The figure shows three views and two pictorial views of one solid part (mm, origin at its lowest corner). Answer the questions. A direction names the side the tool comes from. Coordinates: 2 decimals unless noted, no trailing zeros. Order: outer loops, then holes, each group sorted by start corner. A loop starts at its lowest first (then second) coordinate and runs counter-clockwise, first axis right, second up. Notation, with made-up numbers: M 12,79.25 L 71,79.25 A24 ccw 71,99.25 Z; hole C 27,-15.75 d2. An arc over 180 degrees is marked long. Use a Markdown table: item, result.
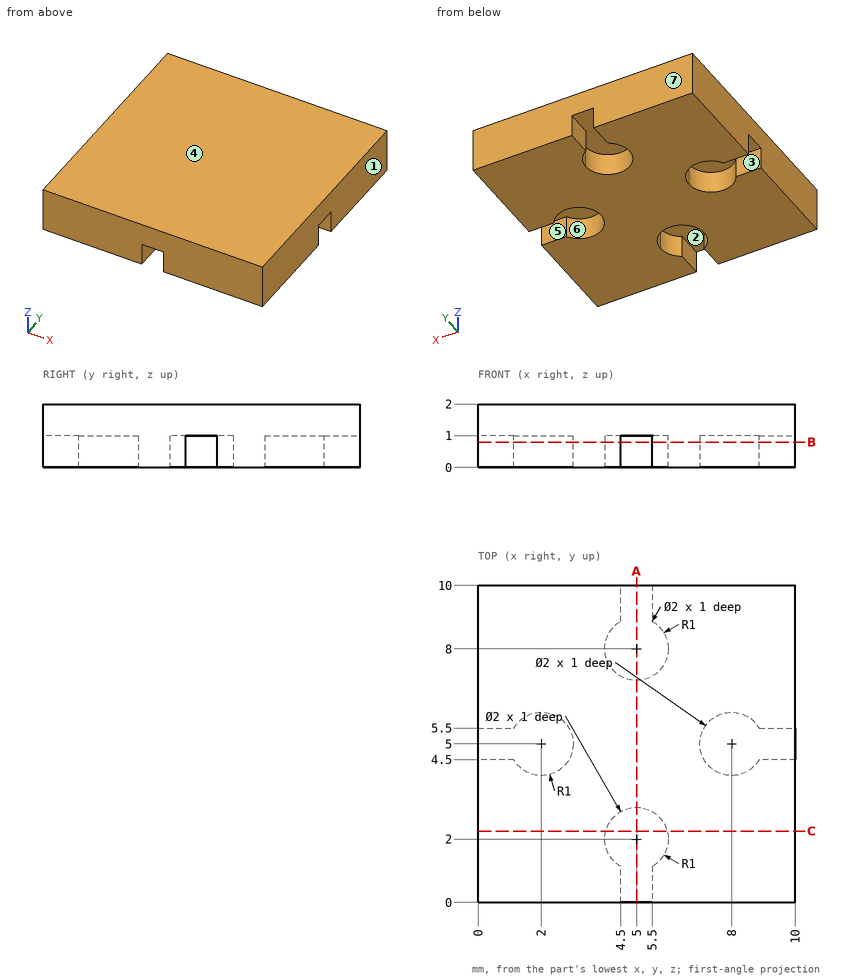
1. For a pull along Y with two mould halves and no side action, classify the marked faces 4, 5, 6 and 7 as +Y half, -Y half, draft (parallel to the pull), parting line (faces both ways), or undercut.
Answers below:
| item | result |
|---|---|
| face 4 | draft |
| face 5 | undercut |
| face 6 | undercut |
| face 7 | +Y half |
2. Section C-C on y = 2.25 is taken. Determine the outline of the cut face in (x, z), then the cut area to 3 significant figures.
Answers below:
| item | result |
|---|---|
| outline | M 0,0 L 4.03,0 L 4.03,1 L 5.97,1 L 5.97,0 L 10,0 L 10,2 L 0,2 Z |
| area | 18.1 mm² |
3. Section B-B on z = 0.8 is taken. Determine the outline of the cut face in (x, y), then the cut area to 3 significant figures.
Answers below:
| item | result |
|---|---|
| outline | M 0,0 L 4.5,0 L 4.5,1.13 A1 cw long 5.5,1.13 L 5.5,0 L 10,0 L 10,4.5 L 8.87,4.5 A1 cw long 8.87,5.5 L 10,5.5 L 10,10 L 5.5,10 L 5.5,8.87 A1 cw long 4.5,8.87 L 4.5,10 L 0,10 L 0,5.5 L 1.13,5.5 A1 cw long 1.13,4.5 L 0,4.5 Z |
| area | 83.3 mm² |
4. For the marked faces 1, 2 and 3, determine the directions among +Z, -Z, +X, -X, +Y, -Y from which every point of the face is accessible in a straight line to the end or side of a thin tool.
Answers below:
| item | result |
|---|---|
| face 1 | +Z, -Z, +X, +Y, -Y |
| face 2 | -Z |
| face 3 | -Z, -X |
5. A flat-ended cylindrical pin translates along its axis: P1, Ø1.2, axis at x = 5, y = 2, coming from the -Z side. Find the tip coordinate at first contact, or state that the pin passes through.
Answers below:
| item | result |
|---|---|
| P1 | z = 1 |
6. Find the intervals of material crossed by probe 1 along X at (y, z) = (9.5, 0.15); probe 2 along X at (y, z) = (2, 0.45); probe 3 along X at (y, z) = (5, 0.35), in increasing order.
Answers below:
| item | result |
|---|---|
| probe 1 | 0 to 4.5, 5.5 to 10 |
| probe 2 | 0 to 4, 6 to 10 |
| probe 3 | 3 to 7 |
7. Section A-A on x = 5 is taken. Determine the outline of the cut face in (y, z).
Answers below:
| item | result |
|---|---|
| outline | M 0,1 L 3,1 L 3,0 L 7,0 L 7,1 L 10,1 L 10,2 L 0,2 Z |
